The model under review builds one solid part; all positions refer to its coordinate system, in mm. A direction names the side the tool comes from. Give positions to 0.01 mm unless a question says otherwise; leave off trailing zeros. Loops run counter-clockwise (first coordinate to the right, second up) from the corner with the lowest first, then second, coordinate; pieces in that order, holes last. Notation, with made-up numbers: (80, 30) - (111, 30) arc R10 cw to (111, 46) - close; hole circle Ø7 at (-37, 22.5). An arc over 180 degrees is marked (long way). Answer as a JSON object with one key per item and string values.
Solid Edge part; units mm, degrees
sketch "Sketch1" plane through (0, 0, 0) normal (0, -1, 0) x (1, 0, 0)
  circle A0 centre (0, 0) radius 19
extrude "Protrusion1" add sketch "Sketch1" against normal blind 225
sketch "Sketch2" plane through (0, 0, 0) normal (0, -1, 0) x (1, 0, 0)
  circle A0 centre (0, 0) radius 10
extrude "ExtrudedCutout_1" cut sketch "Sketch2" against normal blind 40
sketch "Sketch3" plane through (0, 112.5, 0) normal (0, -1, 0) x (1, 0, 0)
  circle A0 centre (0, 0) radius 11
extrude "ExtrudedCutout_3" cut sketch "Sketch3" along normal mid plane 145
hole "Hole_1" at (0, 225, 0) direction (0, -1, 0) diameter 17.835 end up to next thread major 20 thread length 45
sketch "Sketch4" plane through (0, 225, 0) normal (0, 1, 0) x (1, 0, 0)
  line L0 (-2.5, -20) -> (2.5, -20)
  line L1 (2.5, -20) -> (2.5, -17)
  line L2 (2.5, -17) -> (-2.5, -17)
  line L3 (-2.5, -17) -> (-2.5, -20)
extrude "ExtrudedCutout_5" cut sketch "Sketch4" against normal blind 205
fillet "Round_2" radius 5 1 edges at (0, 20, 17)
Q1. Consider section D-D, the plane y = 121. State the section outline as (x, z) points, plus the area to 3 significant figures.
Results:
{"outline": "(-2.5, 17) - (-2.5, 18.83) arc R19 ccw (long way) to (2.5, 18.83) - (2.5, 17) - close; hole circle Ø22 at (0, 0)", "area": "744 mm^2"}
Q2. Clearance check with flat-ended pins moving along their axes: pin 1 Ø1.5 at (x, z) = (13, -2) entering from -Y; pin 2 Ø4 at (x, y) = (1, 135) entering from +Z; pin 3 Ø12 at (x, y) = (-15, 156.5) entering from +Z; pin 4 Ø2 at (y, z) = (109, 18) entering from +X. State where each tip first meets the part, or that it passes through.
Results:
{"pin 1": "stops at y = 0", "pin 2": "stops at z = 18.83", "pin 3": "stops at z = 16.73", "pin 4": "stops at x = 8.49"}
Q3. To check wall thickness, follow probe 1 along Z at (x, y) = (0, 27); probe 2 along Z at (x, y) = (0, 12); probe 3 along X at (y, z) = (215, 0). State the ranges of each line that lie inside material, in increasing order. Write a range as [from, to].
Results:
{"probe 1": "z = [-19, -10], [10, 17]", "probe 2": "z = [-19, -10], [10, 19]", "probe 3": "x = [-19, -8.92], [8.92, 19]"}
Q4. Consider section C-C, the plane x = -4.5. State the section outline as (y, z) points.
Results:
{"outline": "(0, -18.46) - (225, -18.46) - (225, -7.7) - (185, -7.7) - (185, -10.04) - (40, -10.04) - (40, -8.93) - (0, -8.93) - close; (0, 8.93) - (40, 8.93) - (40, 10.04) - (185, 10.04) - (185, 7.7) - (225, 7.7) - (225, 18.46) - (0, 18.46) - close"}
Q5. Consider section B-B, the plane y = 203.5. State the section outline as (x, z) points (1 decimal), plus the area to 3 significant figures.
Results:
{"outline": "(-2.5, 17) - (-2.5, 18.8) arc R19 ccw (long way) to (2.5, 18.8) - (2.5, 17) - close; hole circle Ø17.8 at (0, 0)", "area": "875 mm^2"}
Q6. For faces 1 (the face through (9, 185, 2)), 2 (the face through (-2.17, 19.72, -9.76)), 3 (the face through (0, 126, 17)), list the 3-axis set-ups (+Z, -Z, +X, -X, +Y, -Y) from which the entire face can be reached by the end or side of a thin tool; tool diameter is ignored.
Results:
{"face 1": "none", "face 2": "-Y", "face 3": "+Z, +Y"}
Q7. The part is to be moulded in two halves that separate along Z. For faces 4 (the face through (-8.705, 205.28, -1.933)), 5 (the face through (-4.119, 110.925, -18.548)), 6 (the face through (-8, 0, -8)), say which applies: +Z half, -Z half, draft (parallel to the pull), parting line (faces both ways), or undercut.
Results:
{"face 4": "undercut", "face 5": "parting line", "face 6": "draft"}
Q8. Consider section A-A, the plane z = 0. State the section outline as (x, y) points, plus the area to 3 significant figures.
Results:
{"outline": "(-19, 0) - (-10, 0) - (-10, 40) - (-11, 40) - (-11, 185) - (-8.92, 185) - (-8.92, 225) - (-19, 225) - close; (8.92, 185) - (11, 185) - (11, 40) - (10, 40) - (10, 0) - (19, 0) - (19, 225) - (8.92, 225) - close", "area": "3,850 mm^2"}
